Source: CAD feature listing. Evaluate the final solid. Frame: model axes, mm. A direction names the side the tool comes from. Give positions to 0.01 mm unless a question says otherwise; leave off trailing zeros. Order: outer loops, then holes, each group sorted by start corner. A loop starts at its lowest first (then second) coordinate and runs counter-clockwise, first axis right, second up.
1) First-contact query: P1, Ø1, axis at x = 27, y = 0, coming from the +Z side; P2, Ø2, axis at x = 39.18, z = 0, coming from the -Y side; P3, Ø5.5, axis at x = 0, z = 0, coming from the -Y side. Flat tips, straight axial feed; report the tip coordinate or a pass-through.
2) Access query for faces 1 (the face through (45.962, 0.014, 1.777)), 2 (the face through (33.277, 0.014, 3.787)), 3 (the face through (20.811, 0.014, -16.985)), 4 (the face through (40.402, 0.014, 6.929)). Directions: +Z, -Z, +X, -X, +Y, -Y. A direction counts if a zero-diameter tool reaches every point of the face in a straight line with its end or side. Return the directions, or none.
3) Draft query along X for faces 5 (the face through (42.59, 0.01, 6.16)), 6 (the face through (45.017, 0.014, 3.883)), 7 (the face through (34.05, 0.01, 4.81)). Return one class per face: released by +X, released by -X, zero draft, split by the parting line, or undercut.
4) Material intervals for line 1 (X direction, y = 0.25, z = -3); line 2 (X direction, y = 0.15, z = 6.5); line 3 (X direction, y = -0.5, z = 3), sorted ascending.
5) Section C-C, the plane y = 0.4. Give the number of separate pieces and of enclosed holes in the cut face, plus the area to 3 significant figures.
6) Section B-B, the plane z = -7. Return loops of the section in (x, y).
7) Section D-D, the plane z = -9.75. Return loops of the section in (x, y).
8) Section A-A, the plane x = 0. Return loops of the section in (y, z).
```python
from build123d import *

# Parameters (mm, degrees)
SKETCH1_R           = 1.75
BOSS_EXTRUDE1_DEPTH = 1
CUT_EXTRUDE1_DEPTH  = 10


with BuildPart() as part:
    # Sketch1 → Boss-Extrude1 (new, symmetric)
    with BuildSketch(Plane(origin=(0, 0, 0), x_dir=(1, 0, 0), z_dir=(0, 1, 0))):
        with BuildLine():
            ThreePointArc((-3.468031679, 1.890834809), (-1.940098765, -3.440714574), (3.412697713, -1.988968154))
            ThreePointArc((3.412697713, -1.988968154), (16.498779461, 7.495751106), (32.323208611, 4.210499669))
            ThreePointArc((32.323208611, 4.210499669), (39.413417069, -8.041566659), (45.776010747, 4.603653267))
            ThreePointArc((45.776010747, 4.603653267), (20.398296529, 16.964851371), (-3.468031679, 1.890834809))
        make_face()
        with Locations(Location((0, 0, 0), (0, 0, 270))):
            Circle(SKETCH1_R, mode=Mode.SUBTRACT)
        with Locations(Location((39.178405, 0, 0), (0, 0, 270))):
            Circle(SKETCH1_R, mode=Mode.SUBTRACT)
    extrude(amount=BOSS_EXTRUDE1_DEPTH, both=True)

    # Sketch3 → Cut-Extrude1 (cut)
    with BuildSketch(Plane(origin=(0, 1, 0), x_dir=(1, 0, 0), z_dir=(0, 1, 0))):
        with BuildLine():
            ThreePointArc((32.084811852, 3.795123352), (31.56930529, 2.612207227), (31.24955028, 1.36208951))
            ThreePointArc((31.24955028, 1.36208951), (31.326059207, 1.474902663), (31.450375944, 1.53081127))
            Line((31.450375944, 1.53081127), (33.258253826, 1.797598333))
            ThreePointArc((33.258253826, 1.797598333), (33.381527847, 1.852635734), (33.458211092, 1.963745049))
            ThreePointArc((33.458211092, 1.963745049), (33.46594199, 2.098525734), (33.402466138, 2.217674448))
            Line((33.402466138, 2.217674448), (32.139660471, 3.538628505))
            ThreePointArc((32.139660471, 3.538628505), (32.075896875, 3.659105169), (32.084811852, 3.795123352))
        make_face()
        with BuildLine():
            ThreePointArc((31.236887758, 1.286207175), (31.133405, 0), (31.236887758, -1.286207175))
            ThreePointArc((31.236887758, -1.286207175), (31.272620849, -1.154664142), (31.372048268, -1.061419239))
            Line((31.372048268, -1.061419239), (32.995344721, -0.222070447))
            ThreePointArc((32.995344721, -0.222070447), (33.094068801, -0.129988115), (33.130520001, 0))
            ThreePointArc((33.130520001, 0), (33.094068801, 0.129988115), (32.995344721, 0.222070447))
            Line((32.995344721, 0.222070447), (31.372048268, 1.061419239))
            ThreePointArc((31.372048268, 1.061419239), (31.272620849, 1.154664142), (31.236887758, 1.286207175))
        make_face()
        with BuildLine():
            ThreePointArc((31.24955028, -1.36208951), (31.569305291, -2.61220723), (32.084811854, -3.795123356))
            ThreePointArc((32.084811854, -3.795123356), (32.075896875, -3.659105171), (32.139660471, -3.538628505))
            Line((32.139660471, -3.538628505), (33.402466138, -2.217674449))
            ThreePointArc((33.402466138, -2.217674449), (33.46594199, -2.098525734), (33.458211092, -1.963745049))
            ThreePointArc((33.458211092, -1.963745049), (33.381527847, -1.852635735), (33.258253826, -1.797598333))
            Line((33.258253826, -1.797598333), (31.450375944, -1.53081127))
            ThreePointArc((31.450375944, -1.53081127), (31.326059207, -1.474902664), (31.24955028, -1.36208951))
        make_face()
        with BuildLine():
            ThreePointArc((32.12142724, -3.862782663), (32.829769602, -4.941341274), (33.701436836, -5.892779033))
            ThreePointArc((33.701436836, -5.892779033), (33.648839863, -5.767025378), (33.670029862, -5.632372464))
            Line((33.670029862, -5.632372464), (34.435500154, -3.972959013))
            ThreePointArc((34.435500154, -3.972959013), (34.456849185, -3.839655529), (34.405773951, -3.714687852))
            ThreePointArc((34.405773951, -3.714687852), (34.29716848, -3.634497755), (34.16270317, -3.622469441))
            Line((34.16270317, -3.622469441), (32.366155482, -3.957154626))
            ThreePointArc((32.366155482, -3.957154626), (32.230421073, -3.94464088), (32.12142724, -3.862782663))
        make_face()
        with BuildLine():
            ThreePointArc((33.758037242, -5.944883377), (34.778207068, -6.735004318), (35.911576302, -7.351860666))
            ThreePointArc((35.911576302, -7.351860666), (35.820997033, -7.249998901), (35.79731717, -7.115761472))
            Line((35.79731717, -7.115761472), (35.982501503, -5.297711821))
            ThreePointArc((35.982501503, -5.297711821), (35.959410215, -5.164699069), (35.870525439, -5.063086586))
            ThreePointArc((35.870525439, -5.063086586), (35.741766831, -5.022505549), (35.610681635, -5.054789777))
            Line((35.610681635, -5.054789777), (34.020147957, -5.954678876))
            ThreePointArc((34.020147957, -5.954678876), (33.887704808, -5.98691605), (33.758037242, -5.944883377))
        make_face()
        with BuildLine():
            ThreePointArc((35.982028195, -7.382763732), (37.203474256, -7.798825139), (38.475727347, -8.014254121))
            ThreePointArc((38.475727347, -8.014254121), (38.356981452, -7.947322547), (38.290997808, -7.828047312))
            Line((38.290997808, -7.828047312), (37.875828586, -6.048375351))
            ThreePointArc((37.875828586, -6.048375351), (37.810799277, -5.930067325), (37.693737005, -5.862821327))
            ThreePointArc((37.693737005, -5.862821327), (37.558778252, -5.866246934), (37.445278285, -5.939345207))
            Line((37.445278285, -5.939345207), (36.233117622, -7.306921274))
            ThreePointArc((36.233117622, -7.306921274), (36.118318001, -7.380415969), (35.982028195, -7.382763732))
        make_face()
        with BuildLine():
            ThreePointArc((38.552396173, -8.020607081), (39.842755834, -8.017522246), (41.116024419, -7.808178788))
            ThreePointArc((41.116024419, -7.808178788), (40.981979858, -7.78343048), (40.880842784, -7.692042761))
            Line((40.880842784, -7.692042761), (39.910310035, -6.143603561))
            ThreePointArc((39.910310035, -6.143603561), (39.810389641, -6.052820773), (39.677835385, -6.027228406))
            ThreePointArc((39.677835385, -6.027228406), (39.551301362, -6.07428944), (39.467686107, -6.180280426))
            Line((39.467686107, -6.180280426), (38.765254875, -7.867345373))
            ThreePointArc((38.765254875, -7.867345373), (38.680539103, -7.974133298), (38.552396173, -8.020607081))
        make_face()
        with BuildLine():
            ThreePointArc((41.19060192, -7.7892932), (42.410044691, -7.367396413), (43.546350362, -6.755966128))
            ThreePointArc((43.546350362, -6.755966128), (43.411532943, -6.776082949), (43.286202211, -6.722486022))
            Line((43.286202211, -6.722486022), (41.865478217, -5.573076998))
            ThreePointArc((41.865478217, -5.573076998), (41.741494662, -5.519657171), (41.607812733, -5.538491765))
            ThreePointArc((41.607812733, -5.538491765), (41.503415366, -5.624088433), (41.458745833, -5.751486363))
            Line((41.458745833, -5.751486363), (41.342163355, -7.575220526))
            ThreePointArc((41.342163355, -7.575220526), (41.296711701, -7.703729554), (41.19060192, -7.7892932))
        make_face()
        with BuildLine():
            ThreePointArc((43.610754909, -6.713888537), (44.627135244, -5.918898861), (45.503341649, -4.971639708))
            ThreePointArc((45.503341649, -4.971639708), (45.382360931, -5.034441688), (45.246418071, -5.024443613))
            Line((45.246418071, -5.024443613), (43.529460322, -4.398621067))
            ThreePointArc((43.529460322, -4.398621067), (43.394849148, -4.388353068), (43.274526058, -4.449573603))
            ThreePointArc((43.274526058, -4.449573603), (43.20357842, -4.564430177), (43.202695246, -4.69942951))
            Line((43.202695246, -4.69942951), (43.684595043, -6.462202994))
            ThreePointArc((43.684595043, -6.462202994), (43.683332898, -6.598507176), (43.610754909, -6.713888537))
        make_face()
        with BuildLine():
            ThreePointArc((45.55059401, -4.910929874), (46.253771328, -3.828996777), (46.77492791, -2.648558983))
            ThreePointArc((46.77492791, -2.648558983), (46.68089403, -2.747240553), (46.549070559, -2.781924776))
            Line((46.549070559, -2.781924776), (44.721938068, -2.747506292))
            ThreePointArc((44.721938068, -2.747506292), (44.591286486, -2.781502818), (44.497361108, -2.878475099))
            ThreePointArc((44.497361108, -2.878475099), (44.467551477, -3.010145087), (44.510550368, -3.13811655))
            Line((44.510550368, -3.13811655), (45.538711119, -4.648905496))
            ThreePointArc((45.538711119, -4.648905496), (45.581775256, -4.778234159), (45.55059401, -4.910929874))
        make_face()
        with BuildLine():
            Line((47.052997067, -0.237941224), (45.313687991, -0.798656578))
            ThreePointArc((45.313687991, -0.798656578), (45.201154125, -0.873233578), (45.143804731, -0.995449154))
            ThreePointArc((45.143804731, -0.995449154), (45.158363444, -1.12966407), (45.240584802, -1.236739969))
            Line((45.240584802, -1.236739969), (46.703589337, -2.331826952))
            ThreePointArc((46.703589337, -2.331826952), (46.786313088, -2.440165329), (46.799907556, -2.575795758))
            ThreePointArc((46.799907556, -2.575795758), (47.113681686, -1.324163479), (47.223313041, -0.038465795))
            ThreePointArc((47.223313041, -0.038465795), (47.16641603, -0.162333277), (47.052997067, -0.237941224))
        make_face()
    extrude(amount=-CUT_EXTRUDE1_DEPTH, mode=Mode.SUBTRACT)


solid = part.part
```
From the geometry:
1. P1: stops at z = -6.75
1. P2: passes through
1. P3: stops at y = -1
2. face 1: +X, +Y, -Y
2. face 2: +Y, -Y
2. face 3: -Z, +Y, -Y
2. face 4: +Z, +Y, -Y
3. face 5: undercut
3. face 6: released by +X
3. face 7: released by -X
4. line 1: x = -2.83 to 7.53, 32.65 to 46.64
4. line 2: x = 35.86 to 36.95, 37.98 to 39.33, 40.13 to 41.41, 43.01 to 43.69
4. line 3: x = -2.57 to 2.57, 32.65 to 44.47
5. separate pieces: 1
5. enclosed holes: 2
5. area: 559 mm2
6. outline: (0.08, -1) - (14.63, -1) - (14.63, 1) - (0.08, 1) - close; (26.75, -1) - (43.91, -1) - (43.91, 1) - (26.75, 1) - close
7. outline: (2.8, -1) - (41.19, -1) - (41.19, 1) - (2.8, 1) - close
8. outline: (-1, -6.91) - (1, -6.91) - (1, -1.75) - (-1, -1.75) - close; (-1, 1.75) - (1, 1.75) - (1, 3.95) - (-1, 3.95) - close
